Autodesk Inventor part; units mm, degrees
ref_plane "YZ Plane" through (0, 0, 0) normal (1, 0, 0) x (0, 1, 0)
ref_plane "XZ Plane" through (0, 0, 0) normal (0, 1, 0) x (-1, 0, 0)
ref_plane "XY Plane" through (0, 0, 0) normal (0, 0, 1) x (1, 0, 0)
sketch "Sketch1" plane through (0, 0, 0) normal (0, 1, 0) x (-1, 0, 0)
  line L0 (0, 0) -> (-20, 0)
  line L1 (-20, 0) -> (-20, -40.3)
  line L2 (-20, -40.3) -> (0, -40.3)
  line L3 (0, -40.3) -> (0, 0)
  dimension "d0" = 20
  dimension "d1" = 40.3
extrude "Extrusion1" add sketch "Sketch1" along normal blind 37
sketch "Sketch2" plane through (20, 0, 0) normal (1, 0, 0) x (0, 0, -1)
  line L0 (0, 0) -> (40.3, 0)
  line L1 (40.3, 0) -> (40.3, 37)
  line L2 (21.15, 37) -> (19.15, 37)
  line L3 (19.15, 37) -> (19.15, 0)
  line L4 (19.15, 0) -> (21.15, 0)
  line L5 (21.15, 0) -> (21.15, 37)
  line L6 (0, 37) -> (40.3, 37)
  line L7 (0, 19.5) -> (40.3, 19.5)
  line L8 (40.3, 19.5) -> (40.3, 17.5)
  line L9 (40.3, 17.5) -> (0, 17.5)
  line L10 (0, 17.5) -> (0, 19.5)
  line L11 (0, 0) -> (0, 37)
  point P0 (19.15, 19.5)
  point P1 (19.15, 17.5)
  point P2 (21.15, 17.5)
  point P3 (21.15, 19.5)
  dimension "d5" = 2
  dimension "d6" = 19.15
  dimension "d7" = 0
  dimension "d9" = 2
  dimension "d10" = 17.5
  dimension "d11" = 0
extrude "Extrusion2" add sketch "Sketch2" along normal blind 1 contours L3 L9 L5 L0 | L10 L7 L3 L9 | L3 L7 L5 L9 | L5 L7 L1 L9 | L3 L2 L5 L7
sketch "Sketch3" plane through (0, 0, 0) normal (0, -1, 0) x (1, 0, 0)
  line L0 (0, 0) -> (20, 0)
  line L1 (0, -40.3) -> (0, 0)
  line L2 (20, -40.3) -> (0, -40.3)
  line L3 (20, -21.15) -> (21, -21.15)
  line L4 (21, -19.15) -> (21, -21.15)
  line L5 (20, -19.15) -> (21, -19.15)
  line L6 (21, -19.15) -> (0, -19.15)
  line L7 (0, -19.15) -> (0, -21.15)
  line L8 (0, -21.15) -> (21, -21.15)
  line L9 (21, -21.15) -> (21, -19.15)
  line L10 (0, 0) -> (20, 0)
  line L11 (11, 0) -> (9, 0)
  line L12 (9, 0) -> (9, -40.3)
  line L13 (9, -40.3) -> (11, -40.3)
  line L14 (11, -40.3) -> (11, 0)
  line L15 (9, -40.3) -> (9, 0)
  point P0 (9, -21.15)
  point P1 (11, -21.15)
  point P2 (11, -19.15)
  point P3 (9, -19.15)
  dimension "d14" = 10
  dimension "d15" = 12
  dimension "d16" = 0
extrude "Extrusion3" add sketch "Sketch3" along normal blind 1 contours L0 L14 L6 L12 | L6 L12 L8 L1 | L6 L14 L8 L12 | L6 L5 L4 L3 L8 L14 | L8 L14 L2 L12
sketch "Sketch4" plane through (20, 37, -40.3) normal (0, 0, -1) x (-1, 0, 0)
  line L0 (9, -37) -> (9, -38)
  line L1 (11, -38) -> (9, -38)
  line L2 (11, -37) -> (11, -38)
  line L3 (20, -37) -> (20, 0)
  line L4 (0, 0) -> (20, 0)
  line L5 (0, -17.5) -> (-1, -17.5)
  line L6 (-1, -19.5) -> (-1, -17.5)
  line L7 (0, -19.5) -> (-1, -19.5)
  line L8 (9, -38) -> (11, -38)
  line L9 (11, -38) -> (11, 0)
  line L10 (11, 0) -> (9, 0)
  line L11 (9, 0) -> (9, -38)
  line L12 (-1, -19.5) -> (20, -19.5)
  line L13 (20, -19.5) -> (20, -17.5)
  line L14 (20, -17.5) -> (-1, -17.5)
  line L15 (-1, -17.5) -> (-1, -19.5)
  point P0 (11, -17.5)
  point P1 (9, -17.5)
  point P2 (9, -19.5)
  point P3 (11, -19.5)
extrude "Extrusion4" add sketch "Sketch4" along normal blind 1 contours L11 L12 L9 L2 L1 L0 | L12 L7 L6 L5 L14 L11 | L11 L14 L9 L12 | L11 L4 L9 L14 | L9 L14 L3 L12
sketch "Sketch5" plane through (0, 37, 0) normal (0, 1, 0) x (1, 0, 0)
  line L0 (20, 19.15) -> (21, 19.15)
  line L1 (21, 21.15) -> (21, 19.15)
  line L2 (20, 21.15) -> (21, 21.15)
  line L3 (11, 40.3) -> (11, 41.3)
  line L4 (9, 41.3) -> (11, 41.3)
  line L5 (9, 40.3) -> (9, 41.3)
  line L6 (0, 40.3) -> (0, 0)
  line L7 (0, 0) -> (20, 0)
  line L8 (9, 0) -> (9, 19.15)
  line L9 (11, 41.3) -> (9, 41.3)
  line L10 (9, 41.3) -> (9, 0)
  line L11 (9, 0) -> (11, 0)
  line L12 (11, 0) -> (11, 41.3)
  line L13 (9, 19.15) -> (0, 19.15)
  line L14 (21, 21.15) -> (0, 21.15)
  line L15 (0, 21.15) -> (0, 19.15)
  line L16 (0, 19.15) -> (21, 19.15)
  line L17 (21, 19.15) -> (21, 21.15)
  point P0 (11, 19.15)
  point P1 (11, 21.15)
  point P2 (9, 21.15)
extrude "Extrusion5" add sketch "Sketch5" along normal blind 1 contours L16 L12 L14 L2 L1 L0 | L16 L10 L14 L12 | L12 L7 L8 L16 | L14 L10 L5 L4 L3 L12 | L13 L6 L14 L10
sketch "Sketch6" plane through (0, 0, 0) normal (0, 0, 1) x (1, 0, 0)
  line L0 (9, 0) -> (9, -1)
  line L1 (11, -1) -> (9, -1)
  line L2 (11, 0) -> (11, -1)
  line L3 (20, 17.5) -> (21, 17.5)
  line L4 (21, 19.5) -> (21, 17.5)
  line L5 (20, 19.5) -> (21, 19.5)
  line L6 (11, 37) -> (11, 38)
  line L7 (9, 38) -> (11, 38)
  line L8 (9, 37) -> (9, 38)
  line L9 (0, 0) -> (0, 37)
  line L10 (11, 37) -> (11, 38)
  line L11 (0, -1) -> (9, -1)
  line L12 (11, 38) -> (9, 38)
  line L13 (9, 38) -> (9, -1)
  line L14 (9, -1) -> (11, -1)
  line L15 (11, -1) -> (11, 38)
  line L16 (21, 19.5) -> (21, 17.5)
  line L17 (0, 0) -> (0, 17.5)
  line L18 (21, 19.5) -> (0, 19.5)
  line L19 (0, 19.5) -> (0, 17.5)
  line L20 (0, 17.5) -> (21, 17.5)
  line L21 (21, 17.5) -> (21, 19.5)
  point P0 (11, 17.5)
  point P1 (11, 19.5)
  point P2 (9, 19.5)
  point P3 (9, 17.5)
extrude "Extrusion6" add sketch "Sketch6" along normal blind 1
sketch "Sketch7" plane through (0, 0, -40.3) normal (-1, 0, 0) x (0, 0, 1)
  line L0 (19.15, 0) -> (19.15, -1)
  line L1 (21.15, -1) -> (19.15, -1)
  line L2 (21.15, 0) -> (21.15, -1)
  line L3 (40.3, 17.5) -> (41.3, 17.5)
  line L4 (41.3, 19.5) -> (41.3, 17.5)
  line L5 (40.3, 19.5) -> (41.3, 19.5)
  line L6 (21.15, 37) -> (21.15, 38)
  line L7 (19.15, 38) -> (21.15, 38)
  line L8 (19.15, 37) -> (19.15, 38)
  line L9 (0, 19.5) -> (-1, 19.5)
  line L10 (-1, 17.5) -> (-1, 19.5)
  line L11 (0, 17.5) -> (-1, 17.5)
  line L12 (19.15, -1) -> (21.15, -1)
  line L13 (21.15, -1) -> (19.15, -1)
  line L14 (19.15, -1) -> (19.15, 38)
  line L15 (19.15, 38) -> (21.15, 38)
  line L16 (21.15, 38) -> (21.15, -1)
  line L17 (41.3, 17.5) -> (-1, 17.5)
  line L18 (-1, 17.5) -> (-1, 19.5)
  line L19 (-1, 19.5) -> (41.3, 19.5)
  line L20 (41.3, 19.5) -> (41.3, 17.5)
  point P0 (21.15, 19.5)
  point P1 (19.15, 19.5)
  point P2 (19.15, 17.5)
  point P3 (21.15, 17.5)
extrude "Extrusion7" add sketch "Sketch7" along normal blind 1
sketch "Sketch8" plane through (0, 0, 0) normal (0, -1, 0) x (1, 0, 0)
  circle A0 centre (10, -4) radius 2
  point P0 (0, 0)
  dimension "d27" = 4
extrude "Extrusion8" add sketch "Sketch8" along normal blind 2
sketch "Sketch9" plane through (0, 0, 0) normal (0, 0, 1) x (1, 0, 0)
  line L0 (0, 37) -> (0, 19.5)
  line L1 (0, 0) -> (26.6, 0) construction
  line L2 (0, 26.6) -> (20, 26.6)
  line L3 (20, 19.5) -> (20, 37)
  line L4 (20, 26.6) -> (0, 26.6)
  line L5 (0, 26.6) -> (0, 28.6)
  line L6 (0, 28.6) -> (20, 28.6)
  line L7 (20, 28.6) -> (20, 26.6)
  dimension "d30" = 26.6
  dimension "d32" = 20
  dimension "d33" = 2
extrude "Extrusion9" add sketch "Sketch9" along normal blind 6.7
sketch "Sketch10" plane through (20, 19.5, -40.3) normal (0, 0, -1) x (-1, 0, 0)
  line L0 (0, 0) -> (0, 17.5)
  line L1 (9, 9.1) -> (0, 9.1)
  line L2 (0, 7.1) -> (9, 7.1)
  line L3 (20, 9.1) -> (11, 9.1)
  line L4 (0, 7.1) -> (20, 7.1)
  line L5 (20, 7.1) -> (20, 9.1)
  line L6 (20, 9.1) -> (0, 9.1)
  line L7 (0, 9.1) -> (0, 7.1)
  point P0 (20, -19.5)
extrude "Extrusion10" add sketch "Sketch10" along normal blind 6.7
properties part number "Motor"
Check sheet for the modelled part. Datum: model origin and axes. Units: mm. A direction names the side the tool comes from. Give positions to 0.01 mm unless a question says otherwise; leave off trailing zeros. Write each loop counter-clockwise with the first axis right and the second up, starting at its lowest first coordinate (ties: lowest second). Pieces come first, ordered by that corner, then holes.
Item 1: Cross-section at C-C (z = -4). Enter the section's corners in (x, y), and give its area (3 significant figures).
Item 2: Cross-section at A-A (x = 10). Enter the section's corners in (y, z), and give its area (3 significant figures).
Item 3: Scan lines: L1, parallel to X at y = 35.5, z = -8.5; L2, parallel to Z at x = 6.25, y = 22; L3, parallel to Y at x = 2.25, z = 3. Record each from-to range of solid material in increasing order.
Item 4: Cross-section at D-D (x = 17). Enter the section's corners in (y, z).
Item 5: Gauge pin test, flat ends, axial feed: pin 1 (11 mm diameter, centred on x = 8.5, z = -20.5, fed in from -Y); pin 2 (10 mm diameter, centred on x = 2.5, y = 17, fed in from +Z); pin 3 (5 mm diameter, centred on x = 2, z = -5.5, fed in from +Y). Record the tip position at first contact, or that the pin passes through.
Item 6: Draft check along Y on faces 1 (the face through (10, 16, 1)), 2 (the face through (10, 38, -20)), 3 (the face through (-0.4, 19.5, -33.4)), 4 (the face through (10, -1, -1)). Enter one of: released by +Y, released by -Y, zero draft, split by the parting line, or undercut.
Item 7: Cross-section at B-B (y = 32). Enter the section's corners in (x, z), and give its area (3 significant figures).
Item 8: Access from +Z, -Z, +X, -X, +Y, -Y to the whole of each face (thin tool, end or side, straight path). Record for faces 5 (the face through (5, 37, -31)), 6 (the face through (9.74, -1.208, -5.983)), 7 (the face through (5, 0, -31)), 8 (the face through (-0.4, 19.5, -6.9)).
Report:
1. outline: (-1, 17.5) - (0, 17.5) - (0, 0) - (8, 0) - (8, -2) - (12, -2) - (12, 0) - (20, 0) - (20, 17.5) - (21, 17.5) - (21, 19.5) - (20, 19.5) - (20, 37) - (11, 37) - (11, 38) - (9, 38) - (9, 37) - (0, 37) - (0, 19.5) - (-1, 19.5) - close
1. area: 754 mm2
2. outline: (-2, -6) - (-1, -6) - (-1, -41.3) - (26.6, -41.3) - (26.6, -47) - (28.6, -47) - (28.6, -41.3) - (38, -41.3) - (38, 1) - (28.6, 1) - (28.6, 6.7) - (26.6, 6.7) - (26.6, 1) - (-1, 1) - (-1, -2) - (-2, -2) - close
2. area: 1,680 mm2
3. L1: x = 0 to 20
3. L2: z = -40.3 to 0
3. L3: y = 26.6 to 28.6
4. outline: (-1, -21.15) - (0, -21.15) - (0, -40.3) - (17.5, -40.3) - (17.5, -41.3) - (19.5, -41.3) - (19.5, -40.3) - (26.6, -40.3) - (26.6, -47) - (28.6, -47) - (28.6, -40.3) - (37, -40.3) - (37, -21.15) - (38, -21.15) - (38, -19.15) - (37, -19.15) - (37, 0) - (28.6, 0) - (28.6, 6.7) - (26.6, 6.7) - (26.6, 0) - (19.5, 0) - (19.5, 1) - (17.5, 1) - (17.5, 0) - (0, 0) - (0, -19.15) - (-1, -19.15) - close
5. pin 1: stops at y = -1
5. pin 2: stops at z = 1
5. pin 3: stops at y = 37
6. face 1: zero draft
6. face 2: released by +Y
6. face 3: undercut
6. face 4: released by -Y
7. outline: (-1, -21.15) - (0, -21.15) - (0, -40.3) - (9, -40.3) - (9, -41.3) - (11, -41.3) - (11, -40.3) - (20, -40.3) - (20, -21.15) - (21, -21.15) - (21, -19.15) - (20, -19.15) - (20, 0) - (11, 0) - (11, 1) - (9, 1) - (9, 0) - (0, 0) - (0, -19.15) - (-1, -19.15) - close
7. area: 814 mm2
8. face 5: -Z, -X, +Y
8. face 6: -Y
8. face 7: -Z, -X, -Y
8. face 8: +Z, -X
